Check sheet for the modelled part. Datum: model origin and axes. Units: mm. Give positions to 0.01 mm unless a question says otherwise; leave off trailing zeros. Order: outer loops, then holes, each group sorted by start corner. A loop starts at its lowest first (then second) coordinate and runs counter-clockwise, first axis right, second up. Notation, with made-up numbers: (26, 70.5) -> (66, 70.5) arc R9 ccw to (66, 86.5) -> close; hole circle Ø11 at (13, -6.75). An arc over 180 degrees is marked (long way). Answer in a Markdown table with one row per item. Add a question column.
(1) Cross-section at B-B (y = -14). Record the cut outline in (x, z), then the cut area to 3 significant figures.
(2) Thickness scan on L1, parallel to X at y = 8.5, z = -0.25; L2, parallel to Z at x = 46, y = 14; L3, parallel to Y at x = -11, z = -0.1. Record the ranges inside material, lowest first. Write a range as [from, to].
(3) Cross-section at C-C (x = -25). Record the cut outline in (y, z).
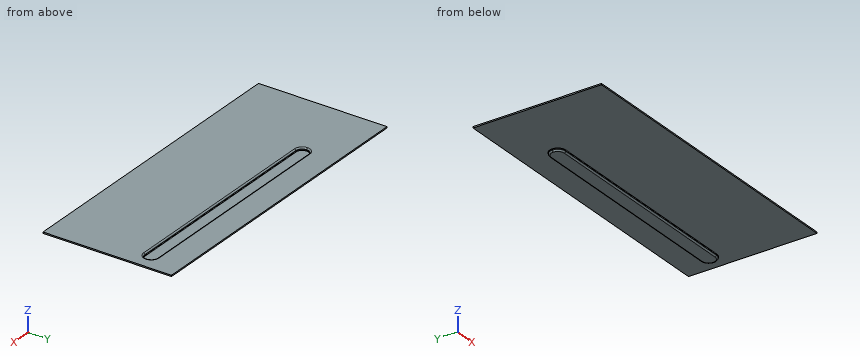
Autodesk Inventor part; units mm, degrees
ref_plane "YZ Plane" through (0, 0, 0) normal (1, 0, 0) x (0, 1, 0)
ref_plane "XZ Plane" through (0, 0, 0) normal (0, 1, 0) x (-1, 0, 0)
ref_plane "XY Plane" through (0, 0, 0) normal (0, 0, 1) x (1, 0, 0)
sketch "Sketch1" plane through (0, 0, 0) normal (0, 0, 1) x (1, 0, 0)
  line L0 (-45, 21.4286) -> (75, 21.4286)
  line L1 (75, 21.4286) -> (75, -28.5714)
  line L2 (75, -28.5714) -> (-45, -28.5714)
  line L3 (-45, -28.5714) -> (-45, 21.4286)
  point P0 (0, 0)
  dimension "d0" = 50
  dimension "d1" = 120
extrude "Plate1" add sketch "Sketch1" along normal blind 0.5
sketch "Sketch2" plane through (0, 0, 0.5) normal (0, 0, 1) x (1, 0, 0)
  line L0 (-19.0588, 11.6471) -> (70.9412, 11.6471)
  line L1 (70.9412, 11.6471) -> (70.9412, 5.6471)
  line L2 (70.9412, 5.6471) -> (-19.0588, 5.6471)
  line L3 (-19.0588, 5.6471) -> (-19.0588, 11.6471)
  point P0 (0, 0)
  point P1 (25.9412, 8.6471)
  dimension "LG_A" = 90
  dimension "LT_A" = 6
  dimension "d5" = 45
  dimension "d6" = 3
extrude "Extrusion1" add sketch "Sketch2" against normal blind 1.4
sketch "Sketch3" plane through (0, 0, 0.5) normal (0, 0, 1) x (1, 0, 0)
  line L0 (-19.0588, 5.6471) -> (-19.0588, 11.6471)
  line L1 (-19.0588, 11.6471) -> (70.9412, 11.6471)
  line L2 (70.9412, 11.6471) -> (70.9412, 5.6471)
  line L3 (70.9412, 5.6471) -> (-19.0588, 5.6471)
  line L4 (-18.5588, 11.1471) -> (70.4412, 11.1471)
  line L5 (70.4412, 11.1471) -> (70.4412, 6.1471)
  line L6 (70.4412, 6.1471) -> (-18.5588, 6.1471)
  line L7 (-18.5588, 6.1471) -> (-18.5588, 11.1471)
  point P0 (0, 0)
  dimension "d9" = 0.5
  dimension "d10" = 0.5
  dimension "d11" = 0.5
  dimension "d12" = 0.5
extrude "Extrusion2" cut sketch "Sketch3" against normal blind 0.9 contours L4 L5 L6 L7
fillet "Fillet1" radius 2.5 4 edges at (-18.5588, 6.1471, 0.05) (-18.5588, 11.1471, 0.05) (70.4412, 11.1471, 0.05) (70.4412, 6.1471, 0.05)
fillet "Fillet2" radius 3 4 edges at (70.9412, 11.6471, -0.45) (70.9412, 5.6471, -0.45) (-19.0588, 11.6471, -0.45) (-19.0588, 5.6471, -0.45)
fillet "Fillet3" radius 0.5 8 edges at (-18.1802, 10.7684, -0.9) (25.9412, 11.6471, -0.9) (70.0625, 10.7684, -0.9) (25.9412, 5.6471, -0.9) (69.709, 10.4149, 0.5) (25.9412, 6.1471, 0.5) (-17.8266, 6.8793, 0.5) (25.9412, 11.1471, 0.5)
fillet "Fillet4" radius 0.2 8 edges at (69.709, 10.4149, -0.4) (25.9412, 6.1471, -0.4) (-17.8266, 6.8793, -0.4) (25.9412, 11.1471, -0.4) (70.0625, 10.7684, 0) (25.9412, 11.6471, 0) (-18.1802, 10.7684, 0) (25.9412, 5.6471, 0)
equation "\"d9\" = Thickness"
equation "\"d10\" = Thickness"
equation "\"d11\" = Thickness"
equation "\"d12\" = Thickness"
equation "\"d2\" = Thickness"
equation "\"GapSize\" = Thickness"
equation "\"BendRadius\" = Thickness"
equation "\"MinimumRemnant\" = 2 * Thickness"
equation "\"BendReliefDepth\" = 0.5 * Thickness"
equation "\"BendReliefWidth\" = Thickness"
equation "\"CornerReliefSize\" = 4 * Thickness"
equation "\"JacobiRadiusSize\" = BendRadius"
equation "\"TransitionRadius\" = BendRadius"
equation "\"d15\" = 0.5 * LT_A - Thickness"
equation "\"d16\" = 0.5 * LT_A"
equation "\"d17\" = Thickness"
properties part number "Amb"
Answer below:
| question | item | result |
|---|---|---|
| 1 | outline | (-45, 0) -> (75, 0) -> (75, 0.5) -> (-45, 0.5) -> close |
| 1 | area | 60.0 mm² |
| 2 | L1 | x = [-19.06, -18.55], [70.43, 70.94] |
| 2 | L2 | z = [0, 0.5] |
| 2 | L3 | y = [5.62, 6.15], [11.15, 11.67] |
| 3 | outline | (-28.57, 0) -> (21.43, 0) -> (21.43, 0.5) -> (-28.57, 0.5) -> close |
